Job drawing, mm, ordinate dimensions from the low corner. One solid piece. A direction names the side the tool comes from. Coordinates: 2 decimals unless noted, no trailing zeros. Write each loop counter-clockwise with the first axis right and the second up, starting at its lowest first coordinate (ties: lowest second). Pieces come first, ordered by that corner, then holes. Notation, with made-up numbers: (-34.75, 10) -> (-21.75, 10) arc R8 cw to (-21.75, 23) -> close; hole circle Ø11 at (-10.5, -33.75). An arc over 180 degrees is marked (long way). One line per question, with ' | ' between items. Start each with the question number.
Item 1: Saw through at D-D (y = 60). List the corners of the cut face in (x, z).
Item 2: Saw through at A-A (x = 93). List the corners of the cut face in (y, z), and give its area (3 significant figures).
Item 3: Saw through at C-C (y = 98). List the corners of the cut face in (x, z).
Item 4: 3-axis set-ups, long thin cutter, end or side, ignore diameter. For the marked faces 1 and 2: which of +Z, -Z, +X, -X, +Y, -Y reach the whole face in a straight line?
Item 5: Saw through at B-B (z = 35). List the corners of the cut face in (x, y).
Item 6: Probe probe 1 along X at (y, z) = (53, 25); probe 2 along Y at (x, z) = (118.5, 38.5); probe 3 along Y at (x, z) = (97.5, 46.5). List the from-to ranges inside material, lowest first. Write a range as [from, to].
Item 7: Two-plate mould, pull along Y, no slides. Class the marked faces 3, 4, 5 and 6: pulls with the +Y half, pulls with the -Y half, needs draft (parallel to the pull), parting line crosses it, or undercut.
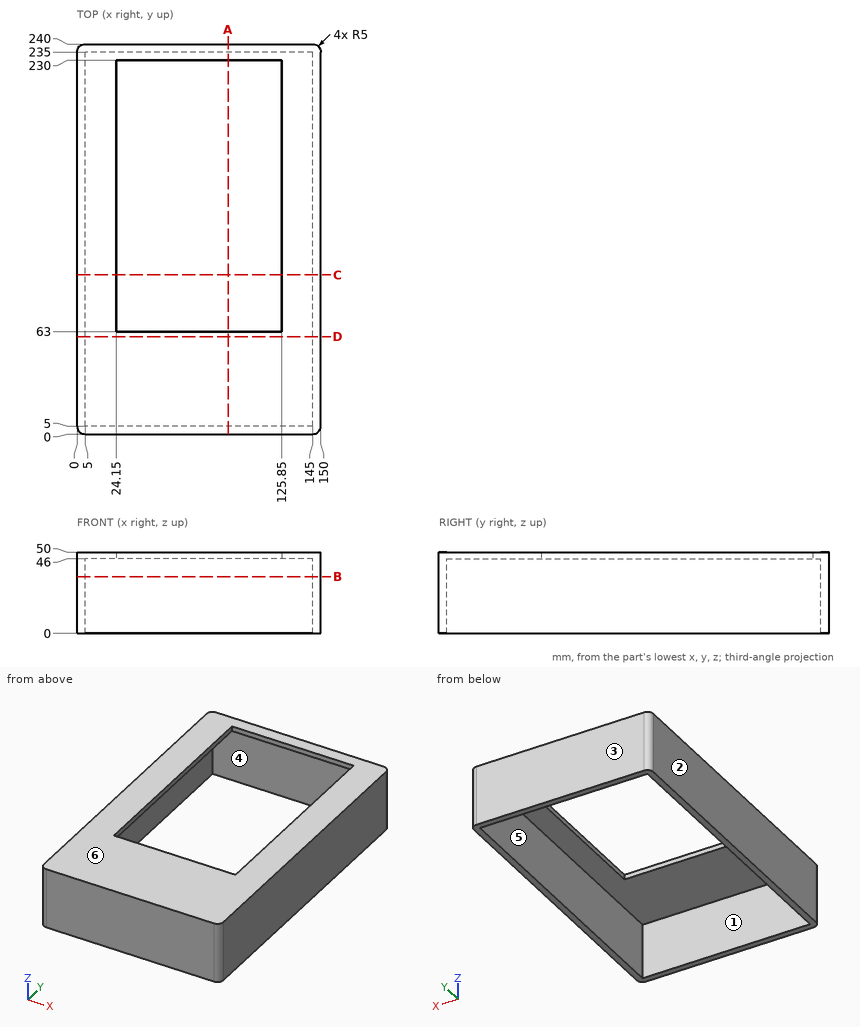
From the geometry:
1) outline: (0, 0) -> (5, 0) -> (5, 46) -> (145, 46) -> (145, 0) -> (150, 0) -> (150, 50) -> (0, 50) -> close
2) outline: (0, 0) -> (5, 0) -> (5, 46) -> (63, 46) -> (63, 50) -> (0, 50) -> close; (230, 46) -> (235, 46) -> (235, 0) -> (240, 0) -> (240, 50) -> (230, 50) -> close | area: 752 mm2
3) outline: (0, 0) -> (5, 0) -> (5, 46) -> (24.15, 46) -> (24.15, 50) -> (0, 50) -> close; (125.85, 46) -> (145, 46) -> (145, 0) -> (150, 0) -> (150, 50) -> (125.85, 50) -> close
4) face 1: -Z | face 2: +Z, -Z, -X, +Y, -Y
5) outline: (0, 5) arc R5 ccw to (5, 0) -> (145, 0) arc R5 ccw to (150, 5) -> (150, 235) arc R5 ccw to (145, 240) -> (5, 240) arc R5 ccw to (0, 235) -> close; hole (5, 5) -> (145, 5) -> (145, 235) -> (5, 235) -> close
6) probe 1: [0, 5], [145, 150] | probe 2: [0, 5], [235, 240] | probe 3: [0, 63], [230, 240]
7) face 3: pulls with the +Y half | face 4: undercut | face 5: undercut | face 6: needs draft
